from build123d import *


with BuildPart() as part:
    # Sketch1 → Revolve1 (revolve)
    with BuildSketch(Plane.XZ.offset(-14.196461829), mode=Mode.PRIVATE) as revolve1_sk:
        Polygon((13.903227856, -1.7), (13.903227856, -7), (15.553227856, -7), (15.553227856, 1.8), (16.303227856, 1.8), (16.303227856, 2.8), (15.203227856, 2.8), (15.203227856, -1.7), align=None)
    revolve(revolve1_sk.sketch.rotate(Axis((12.303227856, 14.196461829, 5), (0, 0, -1)), 180), axis=Axis((12.303227856, 14.196461829, 5), (0, 0, -1)))


solid = part.part
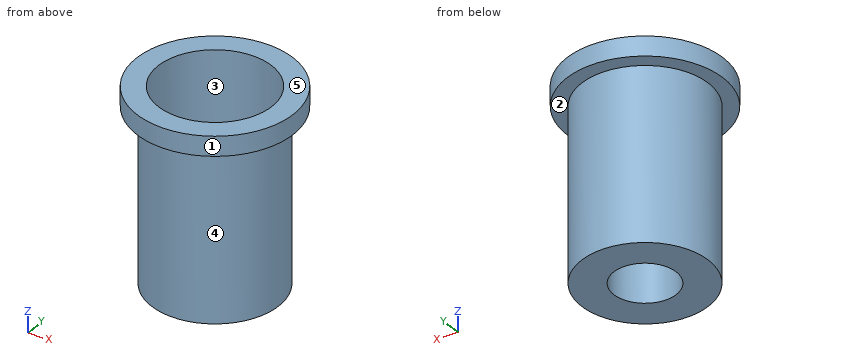
Source: CAD feature listing. Evaluate the final solid. Frame: model axes, mm. Face numbers are marked on the shaded views. A direction names the side the tool comes from. Give positions to 0.01 mm unless a question says otherwise; leave off trailing zeros. Loops run counter-clockwise (first coordinate to the right, second up) from the corner with the lowest first, then second, coordinate; pieces in that order, holes last. Notation, with made-up numbers: (16.5, -39) -> (36.5, -39) arc R24 cw to (36.5, -14) -> close; hole circle Ø3 at (22.25, 16). An arc over 180 degrees is marked (long way). Use a Markdown table: item, result. Add a question column.
1) Section query A-A, the plane y = 13. Return the cut outline in (x, z), then the cut area to 3 significant figures.
2) First-contact query: pin 1 (2 mm diameter, centred on x = 11, z = -1.5, fed in from -Y); pin 2 (1.5 mm diameter, centred on y = 16, z = -2, fed in from -X); pin 3 (3 mm diameter, centred on x = 10.5, z = -3, fed in from +Y); pin 4 (1.9 mm diameter, centred on x = 12.3, y = 14.2, fed in from -Z). Flat tips, straight axial feed; report the tip coordinate or a pass-through.
3) Section query C-C, the plane y = 12. Return the cut outline in (x, z), then the cut area to 3 significant figures.
4) Reachability of the marked faces 1 and 2 from +Z, -Z, +X, -X, +Y, -Y: full face, straight path, thin tool, end or side. Return the list, or none.
5) Section query B-B, the plane x = 13. Return the cut outline in (y, z), then the cut area to 3 significant figures.
6) Pull-direction query (X, two-part tool) for the marked faces 3, 4 and 5; classes: +X half, -X half, draft (parallel to the pull), parting line (faces both ways), or undercut.
7) Section query D-D, the plane x = 9.25. Return the cut outline in (y, z), then the cut area to 3 significant figures.
8) Line query: line 1 along Y through (x, z) = (12.25, 1.75); line 2 along Z through (x, y) = (11.75, 11.5); line 3 along Y through (x, z) = (14.75, 1). Output: solid intervals per line, ascending. Write a range as [from, to].
Numbers:
| question | item | result |
|---|---|---|
| 1 | outline | (8.49, 1.8) -> (9.28, 1.8) -> (9.28, -7) -> (11.24, -7) -> (11.24, -1.7) -> (9.66, -1.7) -> (9.66, 2.8) -> (8.49, 2.8) -> close; (13.37, -7) -> (15.32, -7) -> (15.32, 1.8) -> (16.12, 1.8) -> (16.12, 2.8) -> (14.94, 2.8) -> (14.94, -1.7) -> (13.37, -1.7) -> close |
| 1 | area | 25.8 mm2 |
| 2 | pin 1 | stops at y = 10.96 |
| 2 | pin 2 | stops at x = 9.23 |
| 2 | pin 3 | stops at y = 17.43 |
| 2 | pin 4 | passes through |
| 3 | outline | (8.96, 1.8) -> (9.91, 1.8) -> (9.91, -7) -> (14.7, -7) -> (14.7, 1.8) -> (15.65, 1.8) -> (15.65, 2.8) -> (14.2, 2.8) -> (14.2, -1.7) -> (10.41, -1.7) -> (10.41, 2.8) -> (8.96, 2.8) -> close |
| 3 | area | 31.8 mm2 |
| 4 | face 1 | +Z, -Z |
| 4 | face 2 | -Z |
| 5 | outline | (10.26, 1.8) -> (11.02, 1.8) -> (11.02, -7) -> (12.76, -7) -> (12.76, -1.7) -> (11.38, -1.7) -> (11.38, 2.8) -> (10.26, 2.8) -> close; (15.64, -7) -> (17.37, -7) -> (17.37, 1.8) -> (18.14, 1.8) -> (18.14, 2.8) -> (17.01, 2.8) -> (17.01, -1.7) -> (15.64, -1.7) -> close |
| 5 | area | 23.1 mm2 |
| 6 | face 3 | undercut |
| 6 | face 4 | parting line |
| 6 | face 5 | draft |
| 7 | outline | (11.61, 1.8) -> (13.08, 1.8) -> (13.08, -7) -> (15.31, -7) -> (15.31, 1.8) -> (16.78, 1.8) -> (16.78, 2.8) -> (11.61, 2.8) -> close |
| 7 | area | 24.8 mm2 |
| 8 | line 1 | y = [10.95, 11.3], [17.1, 17.45] |
| 8 | line 2 | z = [-7, -1.7] |
| 8 | line 3 | y = [12.06, 12.64], [15.75, 16.34] |
